```python
from build123d import *

# Parameters (mm, degrees)
SKETCH1_R           = 0.75
BOSS_EXTRUDE1_DEPTH = 2.4
BOSS_EXTRUDE2_START = -8
SKETCH2_R           = 0.75
SKETCH2_R_2         = 0.5
BOSS_EXTRUDE2_DEPTH = 8


with BuildPart() as part:
    # Sketch1 → Boss-Extrude1 (new body)
    with BuildSketch(Plane.XY):
        with BuildLine():
            Line((-0.103544507, 0.982056406), (-0.131068996, 1.243109375))
            ThreePointArc((-0.131068996, 1.243109375), (-0.10199222, 1.373586424), (0, 1.46))
            ThreePointArc((0, 1.46), (0.10199222, 1.373586424), (0.131068996, 1.243109375))
            Line((0.131068996, 1.243109375), (0.103544507, 0.982056406))
            ThreePointArc((0.103544507, 0.982056406), (0.305154282, 0.93916831), (0.493469007, 0.855362256))
            Line((0.493469007, 0.855362256), (0.624644312, 1.082737033))
            ThreePointArc((0.624644312, 1.082737033), (0.724860403, 1.171204283), (0.858166468, 1.181164812))
            ThreePointArc((0.858166468, 1.181164812), (0.889887282, 1.051305237), (0.836718403, 0.928656187))
            Line((0.836718403, 0.928656187), (0.661007538, 0.733638388))
            ThreePointArc((0.661007538, 0.733638388), (0.798904282, 0.580437937), (0.901994132, 0.401948797))
            Line((0.901994132, 0.401948797), (1.141764724, 0.508795946))
            ThreePointArc((1.141764724, 0.508795946), (1.27484099, 0.521461914), (1.388542514, 0.451164812))
            ThreePointArc((1.388542514, 0.451164812), (1.337875649, 0.327461182), (1.222769819, 0.2594879))
            Line((1.222769819, 0.2594879), (0.965988157, 0.204995441))
            ThreePointArc((0.965988157, 0.204995441), (0.9875, 0), (0.965988157, -0.204995441))
            Line((0.965988157, -0.204995441), (1.222769819, -0.2594879))
            ThreePointArc((1.222769819, -0.2594879), (1.337875649, -0.327461182), (1.388542514, -0.451164812))
            ThreePointArc((1.388542514, -0.451164812), (1.27484099, -0.521461914), (1.141764724, -0.508795946))
            Line((1.141764724, -0.508795946), (0.901994132, -0.401948797))
            ThreePointArc((0.901994132, -0.401948797), (0.798904282, -0.580437937), (0.661007538, -0.733638388))
            Line((0.661007538, -0.733638388), (0.836718403, -0.928656187))
            ThreePointArc((0.836718403, -0.928656187), (0.889887282, -1.051305237), (0.858166468, -1.181164812))
            ThreePointArc((0.858166468, -1.181164812), (0.724860403, -1.171204283), (0.624644312, -1.082737033))
            Line((0.624644312, -1.082737033), (0.493469007, -0.855362256))
            ThreePointArc((0.493469007, -0.855362256), (0.305154282, -0.93916831), (0.103544507, -0.982056406))
            Line((0.103544507, -0.982056406), (0.131068996, -1.243109375))
            ThreePointArc((0.131068996, -1.243109375), (0.10199222, -1.373586424), (0, -1.46))
            ThreePointArc((0, -1.46), (-0.10199222, -1.373586424), (-0.131068996, -1.243109375))
            Line((-0.131068996, -1.243109375), (-0.103544507, -0.982056406))
            ThreePointArc((-0.103544507, -0.982056406), (-0.305154282, -0.93916831), (-0.493469007, -0.855362256))
            Line((-0.493469007, -0.855362256), (-0.624644312, -1.082737033))
            ThreePointArc((-0.624644312, -1.082737033), (-0.724860403, -1.171204283), (-0.858166468, -1.181164812))
            ThreePointArc((-0.858166468, -1.181164812), (-0.889887282, -1.051305237), (-0.836718403, -0.928656187))
            Line((-0.836718403, -0.928656187), (-0.661007538, -0.733638388))
            ThreePointArc((-0.661007538, -0.733638388), (-0.798904282, -0.580437937), (-0.901994132, -0.401948797))
            Line((-0.901994132, -0.401948797), (-1.141764724, -0.508795946))
            ThreePointArc((-1.141764724, -0.508795946), (-1.27484099, -0.521461914), (-1.388542514, -0.451164812))
            ThreePointArc((-1.388542514, -0.451164812), (-1.337875649, -0.327461182), (-1.222769819, -0.2594879))
            Line((-1.222769819, -0.2594879), (-0.965988157, -0.204995441))
            ThreePointArc((-0.965988157, -0.204995441), (-0.9875, 0), (-0.965988157, 0.204995441))
            Line((-0.965988157, 0.204995441), (-1.222769819, 0.2594879))
            ThreePointArc((-1.222769819, 0.2594879), (-1.337875649, 0.327461182), (-1.388542514, 0.451164812))
            ThreePointArc((-1.388542514, 0.451164812), (-1.27484099, 0.521461914), (-1.141764724, 0.508795946))
            Line((-1.141764724, 0.508795946), (-0.901994132, 0.401948797))
            ThreePointArc((-0.901994132, 0.401948797), (-0.798904282, 0.580437937), (-0.661007538, 0.733638388))
            Line((-0.661007538, 0.733638388), (-0.836718403, 0.928656187))
            ThreePointArc((-0.836718403, 0.928656187), (-0.889887282, 1.051305237), (-0.858166468, 1.181164812))
            ThreePointArc((-0.858166468, 1.181164812), (-0.724860403, 1.171204283), (-0.624644312, 1.082737033))
            Line((-0.624644312, 1.082737033), (-0.493469007, 0.855362256))
            ThreePointArc((-0.493469007, 0.855362256), (-0.305154282, 0.93916831), (-0.103544507, 0.982056406))
        make_face()
        Circle(SKETCH1_R, mode=Mode.SUBTRACT)
    extrude(amount=BOSS_EXTRUDE1_DEPTH)

    # Sketch2 → Boss-Extrude2 (add)
    with BuildSketch(Plane.XY.offset(2.4).offset(BOSS_EXTRUDE2_START)):
        Circle(SKETCH2_R)
        Circle(SKETCH2_R_2, mode=Mode.SUBTRACT)
    extrude(amount=BOSS_EXTRUDE2_DEPTH)


solid = part.part
```
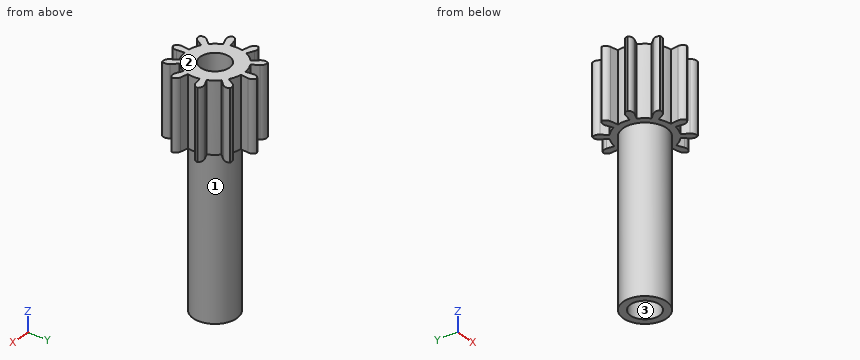
Verification items for the finished model (mm, model axes). Face numbers are marked on the shaded views. Give positions to 0.01 mm unless a question says otherwise; leave off trailing zeros. Order: outer loops, then holes, each group sorted by start corner. A loop starts at its lowest first (then second) coordinate and runs counter-clockwise, first axis right, second up. Notation, with made-up numbers: (18.5, 80) -> (25.5, 80) arc R23 ccw to (25.5, 99) -> close; hole circle Ø4 at (64.25, 16). An arc over 180 degrees is marked (long way). Use a Markdown table: item, result.
1) Section check A-A, the plane y = 0. Record the boundary of the cut face in (x, z), then the cut area to 3 significant figures.
Results:
| item | result |
|---|---|
| outline | (-0.99, 0) -> (-0.75, 0) -> (-0.75, -5.6) -> (-0.5, -5.6) -> (-0.5, 2.4) -> (-0.99, 2.4) -> close; (0.5, -5.6) -> (0.75, -5.6) -> (0.75, 0) -> (0.99, 0) -> (0.99, 2.4) -> (0.5, 2.4) -> close |
| area | 5.14 mm² |
2) Section check B-B, the plane x = 0.4. Record the boundary of the cut face in (y, z).
Results:
| item | result |
|---|---|
| outline | (-0.9, 0) -> (-0.63, 0) -> (-0.63, -5.6) -> (-0.3, -5.6) -> (-0.3, 2.4) -> (-0.9, 2.4) -> close; (0.3, -5.6) -> (0.63, -5.6) -> (0.63, 0) -> (0.9, 0) -> (0.9, 2.4) -> (0.3, 2.4) -> close |
3) Mould release check, pull along X, two halves, no side actions. Record for the marked faces 1, 2 and 3: pulls with the +X half, pulls with the -X half, needs draft (parallel to the pull), parting line crosses it, or undercut.
Results:
| item | result |
|---|---|
| face 1 | parting line crosses it |
| face 2 | needs draft |
| face 3 | undercut |
4) Material ranges on probe 1 along Y at (x, z) = (0, -2); probe 2 along X at (y, z) = (-1.3, 0.5); probe 3 along Z at (x, y) = (-0.95, -0.35), recorded low to high.
Results:
| item | result |
|---|---|
| probe 1 | -0.75 to -0.5, 0.5 to 0.75 |
| probe 2 | -0.13 to 0.13 |
| probe 3 | 0 to 2.4 |
5) Section check C-C, the plane z = -3.25. Record the boundary of the cut face in (x, y), then the cut area to 3 significant figures.
Results:
| item | result |
|---|---|
| outline | circle Ø1.5 at (0, 0); hole circle Ø1 at (0, 0) |
| area | 0.982 mm² |
